```python
from build123d import *

# Parameters (mm, degrees)
SKETCH1_W           = 42
SKETCH1_H           = 42
BOSS_EXTRUDE1_DEPTH = 33
SKETCH2_R           = 11
BOSS_EXTRUDE2_DEPTH = 2
SKETCH3_R           = 2.5
BOSS_EXTRUDE3_DEPTH = 18
SKETCH4_R           = 1.5
CUT_EXTRUDE1_DEPTH  = 5
CHAMFER1_SIZE       = 5
CHAMFER2_SIZE       = 0.5
FILLET1_R           = 0.5
FILLET2_R           = 0.5


with BuildPart() as part:
    # Sketch1 → Boss-Extrude1 (new body)
    with BuildSketch(Plane(origin=(0, 0, 0), x_dir=(1, 0, 0), z_dir=(0, 1, 0))):
        Rectangle(SKETCH1_W, SKETCH1_H)
    extrude(amount=BOSS_EXTRUDE1_DEPTH)

    # Sketch2 → Boss-Extrude2 (add)
    with BuildSketch(Plane(origin=(0, 33, 0), x_dir=(1, 0, 0), z_dir=(0, 1, 0))):
        with Locations(Location((0, 0, 0), (0, 0, 270))):
            Circle(SKETCH2_R)
    extrude(amount=BOSS_EXTRUDE2_DEPTH)

    # Sketch3 → Boss-Extrude3 (add)
    with BuildSketch(Plane(origin=(0, 35, 0), x_dir=(1, 0, 0), z_dir=(0, 1, 0))):
        with Locations(Location((0, 0, 0), (0, 0, 270))):
            Circle(SKETCH3_R)
    extrude(amount=BOSS_EXTRUDE3_DEPTH)

    # Sketch4 → Cut-Extrude1 (cut)
    with BuildSketch(Plane(origin=(0, 33, 0), x_dir=(1, 0, 0), z_dir=(0, 1, 0))):
        with Locations(Location((-15.5, 15.5, 0), (0, 0, 270))):
            Circle(SKETCH4_R)
        with Locations(Location((15.5, 15.5, 0), (0, 0, 270))):
            Circle(SKETCH4_R)
        with Locations(Location((15.5, -15.5, 0), (0, 0, 270))):
            Circle(SKETCH4_R)
        with Locations(Location((-15.5, -15.5, 0), (0, 0, 270))):
            Circle(SKETCH4_R)
    extrude(amount=-CUT_EXTRUDE1_DEPTH, mode=Mode.SUBTRACT)

    # Chamfer1
    chamfer1_edges = [part.edges().sort_by_distance(p)[0] for p in [
        (-21, 16.5, -21),
        (21, 16.5, -21),
        (21, 16.5, 21),
        (-21, 16.5, 21),
    ]]
    chamfer(chamfer1_edges, length=CHAMFER1_SIZE)

    # Chamfer2
    chamfer2_edges = [part.edges().sort_by_distance(p)[0] for p in [
        (-15.5, 33, -17),
        (15.5, 33, -17),
        (15.5, 33, 14),
        (-15.5, 33, 14),
    ]]
    chamfer(chamfer2_edges, length=CHAMFER2_SIZE)

    # Fillet1
    fillet1_edges = [part.edges().sort_by_distance(p)[0] for p in [
        (0, 0, 21),
        (0, 33, 21),
        (-21, 0, 0),
        (0, 0, -21),
        (21, 0, 0),
        (18.5, 0, 18.5),
        (18.5, 0, -18.5),
        (-18.5, 0, -18.5),
        (-18.5, 0, 18.5),
        (-21, 33, 0),
        (21, 33, 0),
        (0, 33, -21),
        (18.5, 33, 18.5),
        (18.5, 33, -18.5),
        (-18.5, 33, -18.5),
        (-18.5, 33, 18.5),
    ]]
    fillet(fillet1_edges, radius=FILLET1_R)

    # Fillet2
    fillet2_edges = [part.edges().sort_by_distance(p)[0] for p in [
        (0, 35, -11),
    ]]
    fillet(fillet2_edges, radius=FILLET2_R)


solid = part.part
```
Can you work these out from the model? Positions are in its coordinate system, mm. A direction names the side the tool comes from. Round coordinates to 2 decimals unless told otherwise and drop trailing zeros. Loops run counter-clockwise (first coordinate to the right, second up) from the corner with the lowest first, then second, coordinate; pieces in that order, holes last. Notation, with made-up numbers: M -24.5,28.25 L 11.5,28.25 A21 ccw 11.5,47.25 Z; hole C 54.5,55 d8. An arc over 180 degrees is marked long. Write item = value, one per line. Start each with the question number.
(1) I'm going to push flat-ended pins straight in: P1, Ø3, axis at x = -16.5, z = -12, coming from the +Y side; P2, Ø23, axis at x = -5, z = -4.5, coming from the +Y side; P3, Ø3.5, axis at x = -15.5, z = -15.5, coming from the +Y side; P4, Ø0.9, axis at x = 16, z = 15.5, coming from the +Y side. Where does each tip first touch, or does it pass through?
(2) If we mould it in two halves opening along X, with no side actions, what happens to faces 3 (the face through (-2, 35, 2)), 4 (the face through (18.429, 32.857, -18.359)), 5 (the face through (-15, 28, 15))? For each: released by +X, released by -X, zero draft, split by the parting line, or undercut.
(3) Suppose I cut it at A-A on x = 12.5. Write out the boundary of the cut face in (y, z).
(4) Suppose I cut it at C-C on y = 39.5. Write out the boundary of the cut face in (x, z).
(5) Suppose I cut it at D-D on z = 12.5. Write out the boundary of the cut face in (x, y).
(6) Which directions (+Z, -Z, +X, -X, +Y, -Y) give clear straight access to the entire face, cutting with the end or side of a thin tool? Please do faces 1 (the face through (-10.74, 33.74, -2.38)), 2 (the face through (0, 16, 21)).
(7) Suppose I cut it at B-B on z = 0. Write out the boundary of the cut face in (x, y), plus the area to 3 significant figures.
(8) I need wall thicknesses on line 1 along X through (y, z) = (30.05, -15.5); line 2 along X through (y, z) = (29, 15); line 3 along Y through (x, z) = (-7, 19). Which ranges of each line are inside material? Lowest first, please.
Answer block:
q1.P1 = 33
q1.P2 = 53
q1.P3 = 32.75
q1.P4 = 28
q2.face_3 = zero draft
q2.face_4 = released by +X
q2.face_5 = undercut
q3.outline = M 0,-20.5 A0.5 ccw 0.5,-21 L 32.5,-21 A0.5 ccw 33,-20.5 L 33,20.5 A0.5 ccw 32.5,21 L 0.5,21 A0.5 ccw 0,20.5 Z
q4.outline = C 0,0 d5
q5.outline = M -21,0.5 A0.5 ccw -20.5,0 L 20.5,0 A0.5 ccw 21,0.5 L 21,32.5 A0.5 ccw 20.5,33 L -20.5,33 A0.5 ccw -21,32.5 Z
q6.face_1 = +Y
q6.face_2 = +Z, +X, -X, +Y, -Y
q7.outline = M -21,0.5 A0.5 ccw -20.5,0 L 20.5,0 A0.5 ccw 21,0.5 L 21,32.5 A0.5 ccw 20.5,33 L 11,33 L 11,34.5 A0.5 ccw 10.5,35 L 2.5,35 L 2.5,53 L -2.5,53 L -2.5,35 L -10.5,35 A0.5 ccw -11,34.5 L -11,33 L -20.5,33 A0.5 ccw -21,32.5 Z
q7.area = 1,520 mm²
q8.line_1 = -21 to -17, -14 to 14, 17 to 21
q8.line_2 = -21 to -16.91, -14.09 to 14.09, 16.91 to 21
q8.line_3 = 0 to 33
